Can you work these out from the model? Positions are in its coordinate system, mm. A direction names the side the tool comes from. Round coordinates to 2 decimals unless told otherwise and drop trailing zeros. Order: outer loops, then holes, each group sorted by start corner. A loop starts at its lowest first (then second) coordinate and runs counter-clockwise, first axis right, second up. Notation, with made-up numbers: (-23, -19.75) - (-3, -19.75) arc R29 ccw to (-3, 5.25) - close; hole circle Ø2 at (15, 85). An arc over 180 degrees is marked (long way). Write item = value, one per line.
from build123d import *

# Parameters (mm, degrees)
PAD_DEPTH = 2


with BuildPart() as part:
    # Sketch → Pad (new body)
    with BuildSketch(Plane.XY):
        with BuildLine():
            ThreePointArc((-15, 0), (0, -15), (15, 0))
            Line((15, 0), (15, 30))
            ThreePointArc((15, 30), (0, 45), (-15, 30))
            Line((-15, 30), (-15, 0))
        make_face()
        with BuildLine():
            ThreePointArc((-7, -10.954451), (6.244998, -11.401754), (13, 0))
            Line((13, 30), (13, 0))
            ThreePointArc((13, 30), (6.244998, 41.401754), (-7, 40.954451))
            Line((-7, 40.954451), (-7, 36.801294))
            ThreePointArc((-7, 36.801294), (-9.043716, 33.669986), (-9.76, 30))
            Line((-9.76, 30), (-9.76, 0))
            ThreePointArc((-9.76, 0), (-9.043716, -3.669986), (-7, -6.801294))
            Line((-7, -10.954451), (-7, -6.801294))
        make_face(mode=Mode.SUBTRACT)
    extrude(amount=PAD_DEPTH)


solid = part.part
(1) Will this pin go through, and if not, where does the flat tip stop? P1, Ø1, axis at y = -9, z = 1, coming from the +X side.
Computed:
P1 = 12.36
(2) If we section it at A-A (z = 1.15): Write out the boundary of the cut face in (x, y), plus the area to 3 significant figures.
Computed:
outline = (-15, 0) arc R15 ccw to (15, 0) - (15, 30) arc R15 ccw to (-15, 30) - close; hole (-9.76, 0) arc R9.76 ccw to (-7, -6.8) - (-7, -10.95) arc R13 ccw to (13, 0) - (13, 30) arc R13 ccw to (-7, 40.95) - (-7, 36.8) arc R9.76 ccw to (-9.76, 30) - close
area = 460 mm^2
(3) Thinking about a two-plate mould opening in Y: for faces 1 (the face through (-15, 15, 1)), 2 (the face through (-9.063, -3.621, 0.986)), 3 (the face through (0, -15, 1)), which applies, +Y half, -Y half, draft (parallel to the pull), parting line (faces both ways), or undercut?
Computed:
face_1 = draft
face_2 = undercut
face_3 = -Y half
(4) If I drill on line 1 (X direction, y = 22, z = 1.1); line 2 (Y direction, x = 11, z = 1); line 3 (Y direction, x = -3.5, z = 1.8), over which ranges is the centre line in solid material (lowest first)? Write a range as from..to.
Computed:
line_1 = -15..-9.76, 13..15
line_2 = -10.2..-6.93, 36.93..40.2
line_3 = -14.59..-12.52, 42.52..44.59
(5) If we section it at C-C (y = 14.5): Write out the boundary of the cut face in (x, z).
Computed:
outline = (-15, 0) - (-9.76, 0) - (-9.76, 2) - (-15, 2) - close; (13, 0) - (15, 0) - (15, 2) - (13, 2) - close
(6) If we section it at B-B (x = 0): Write out the boundary of the cut face in (y, z).
Computed:
outline = (-15, 0) - (-13, 0) - (-13, 2) - (-15, 2) - close; (43, 0) - (45, 0) - (45, 2) - (43, 2) - close
(7) On a 3-axis mill with a long thin cutter (end or side, diameter ignored), from which of +Z, -Z, +X, -X, +Y, -Y can I reach the whole of each face in a straight line? I mean faces 4 (the face through (0, 45, 1)), 5 (the face through (6.415, 41.307, 0.986)). Say none if no direction works.
Computed:
face_4 = +Z, -Z, +Y
face_5 = +Z, -Z
